The listing builds one solid part. Answer for the finished solid, in the listing's coordinates (mm). Round coordinates to 2 decimals unless told otherwise and drop trailing zeros. Order: outer loops, then holes, each group sorted by start corner. A loop starts at its lowest first (then second) coordinate and runs counter-clockwise, first axis right, second up. Notation, with made-up numbers: M 29.5,21 L 56.5,21 A21 ccw 56.5,41 Z; hole C -20.75,-31 d11. An arc over 180 degrees is marked long. Put each result on its own line as item: value. Start each with the question number.
1. The part is cut by section C-C (y = 2.45). Give the vertices of the cut face in (x, z) (3 decimals), then the cut area to 3 significant figures.
2. Each of these flat-tipped pins is pushed along its axis until it touches: pin 1 Ø1 at (x, y) = (4, 2.5) entering from +Z; pin 2 Ø2 at (x, z) = (-1, -10) entering from -Y. Where does it stop, or does it pass through?
3. The part is cut by section B-B (x = 0). Give the vertices of the cut face in (y, z).
4. Consider line 1 (X direction, y = 1.1, z = 0) (3 decimals); line 2 (Z direction, x = 7.8, y = 0.7) (3 decimals); line 3 (Z direction, x = -2, y = 1.45). Determine where each line is inside the solid, lowest interval first.
5. The mould has two halves that part along X. Classify faces 1 (the face through (0, 3, -4)), 2 (the face through (6.476, 1.479, -0.058)), 3 (the face through (-8.44, 1.48, 12.65)), 4 (the face through (8.44, 1.48, -12.65)): +X half, -X half, draft (parallel to the pull), parting line (faces both ways), or undercut.
6. The part is cut by section A-A (z = 0). Give the vertices of the cut face in (x, y) (3 decimals).
7. The part is cut by section D-D (x = 7.8). Give the vertices of the cut face in (y, z) (3 decimals), then the cut area to 3 significant figures.
from build123d import *

# Parameters (mm, degrees)
SKETCH1_R           = 1.325
SKETCH1_R_2         = 2.85
BOSS_EXTRUDE1_DEPTH = 3


with BuildPart() as part:
    # Sketch1 → Boss-Extrude1 (new body)
    with BuildSketch(Plane(origin=(0, 0, 0), x_dir=(1, 0, 0), z_dir=(0, 1, 0))):
        with BuildLine():
            Line((-1.45, 15.5), (1.45, 15.5))
            ThreePointArc((1.45, 15.5), (8.521067812, 12.571067812), (11.45, 5.5))
            Line((11.45, 5.5), (11.45, -5.5))
            ThreePointArc((11.45, -5.5), (8.521067812, -12.571067812), (1.45, -15.5))
            Line((1.45, -15.5), (-1.45, -15.5))
            ThreePointArc((-1.45, -15.5), (-8.521067812, -12.571067812), (-11.45, -5.5))
            Line((-11.45, -5.5), (-11.45, 5.5))
            ThreePointArc((-11.45, 5.5), (-8.521067812, 12.571067812), (-1.45, 15.5))
        make_face()
        with Locations((7.8, 0)):
            Circle(SKETCH1_R, mode=Mode.SUBTRACT)
        with Locations((-7.8, 0)):
            Circle(SKETCH1_R, mode=Mode.SUBTRACT)
        Circle(SKETCH1_R_2, mode=Mode.SUBTRACT)
    extrude(amount=BOSS_EXTRUDE1_DEPTH)


solid = part.part
Resolved:
1. outline: M -11.45,-5.5 A10 ccw -1.45,-15.5 L 1.45,-15.5 A10 ccw 11.45,-5.5 L 11.45,5.5 A10 ccw 1.45,15.5 L -1.45,15.5 A10 ccw -11.45,5.5 Z; hole C -7.8,0 d2.65; hole C 0,0 d5.7; hole C 7.8,0 d2.65
1. area: 588 mm2
2. pin 1: z = 15.29
2. pin 2: y = 0
3. outline: M 0,-15.5 L 3,-15.5 L 3,-2.85 L 0,-2.85 Z; M 0,2.85 L 3,2.85 L 3,15.5 L 0,15.5 Z
4. line 1: -11.45 to -9.125, -6.475 to -2.85, 2.85 to 6.475, 9.125 to 11.45
4. line 2: -13.225 to -1.325, 1.325 to 13.225
4. line 3: -15.48 to -2.03, 2.03 to 15.48
5. face 1: draft
5. face 2: undercut
5. face 3: -X half
5. face 4: +X half
6. outline: M -11.45,0 L -9.125,0 L -9.125,3 L -11.45,3 Z; M -6.475,0 L -2.85,0 L -2.85,3 L -6.475,3 Z; M 2.85,0 L 6.475,0 L 6.475,3 L 2.85,3 Z; M 9.125,0 L 11.45,0 L 11.45,3 L 9.125,3 Z
7. outline: M 0,-13.225 L 3,-13.225 L 3,-1.325 L 0,-1.325 Z; M 0,1.325 L 3,1.325 L 3,13.225 L 0,13.225 Z
7. area: 71.4 mm2
